from build123d import *

# Parameters (mm, degrees)
SKETCH1_R           = 10
BOSS_EXTRUDE1_DEPTH = 20
BOSS_EXTRUDE2_DEPTH = 20
CUT_EXTRUDE1_DEPTH  = 15
SKETCH5_R           = 20
BOSS_EXTRUDE3_DEPTH = 5


with BuildPart() as part:
    # Sketch1 → Boss-Extrude1 (new body)
    with BuildSketch(Plane.XY):
        with BuildLine():
            Line((-71.370560529, 20), (276.629439471, 20))
            ThreePointArc((276.629439471, 20), (296.629439471, 0), (276.629439471, -20))
            Line((276.629439471, -20), (-71.370560529, -20))
            ThreePointArc((-71.370560529, -20), (-91.370560529, 0), (-71.370560529, 20))
        make_face()
        with Locations((-71.370560529, 0)):
            Circle(SKETCH1_R, mode=Mode.SUBTRACT)
        with Locations((276.629439471, 0)):
            Circle(SKETCH1_R, mode=Mode.SUBTRACT)
    extrude(amount=BOSS_EXTRUDE1_DEPTH)

    # Sketch2 → Boss-Extrude2 (add)
    with BuildSketch(Plane(origin=(0, 0, 0), x_dir=(-1, 0, 0), z_dir=(0, 0, -1))):
        with BuildLine():
            Line((71.370560529, -20), (71.370560529, -25))
            ThreePointArc((71.370560529, -25), (64.900084402, -24.148145657), (58.870560529, -21.650635095))
            Line((58.870560529, -21.650635095), (62.564306071, -17.956889553))
            ThreePointArc((62.564306071, -17.956889553), (66.850482602, -19.482527955), (71.370560529, -20))
        make_face()
    extrude(amount=BOSS_EXTRUDE2_DEPTH)

    # Sketch6 → Cut-Extrude1 (cut)
    with BuildSketch(Plane.XY.offset(20)):
        with BuildLine():
            ThreePointArc((-88.39401573, 13.427541495), (-86.445115044, 11.855559488), (-84.410885886, 10.395678313))
            ThreePointArc((-84.410885886, 10.395678313), (-82.694985814, 12.298884863), (-80.712431568, 13.922457124))
            ThreePointArc((-80.712431568, 13.922457124), (-81.560998495, 16.374699705), (-82.281198511, 18.867664093))
            ThreePointArc((-82.281198511, 18.867664093), (-79.798448631, 20.149575363), (-77.17323964, 21.106456352))
            ThreePointArc((-77.17323964, 21.106456352), (-76.520533705, 18.689161112), (-75.73290437, 16.312402533))
            ThreePointArc((-75.73290437, 16.312402533), (-73.22603531, 16.843548219), (-70.667803401, 16.991729622))
            ThreePointArc((-70.667803401, 16.991729622), (-69.912916442, 19.47441067), (-69.030242792, 21.914584175))
            ThreePointArc((-69.030242792, 21.914584175), (-66.268167407, 21.492348412), (-63.581888186, 20.723422265))
            ThreePointArc((-63.581888186, 20.723422265), (-64.474688485, 18.384138413), (-65.234506609, 15.998343424))
            ThreePointArc((-65.234506609, 15.998343424), (-62.894207335, 14.954548647), (-60.737455402, 13.570738932))
            ThreePointArc((-60.737455402, 13.570738932), (-58.667455717, 15.135558669), (-56.519059735, 16.59087795))
            ThreePointArc((-56.519059735, 16.59087795), (-54.532677763, 14.625774866), (-52.811395672, 12.424745236))
            ThreePointArc((-52.811395672, 12.424745236), (-54.908682835, 11.056999694), (-56.925723719, 9.57346089))
            ThreePointArc((-56.925723719, 9.57346089), (-55.645909011, 7.353419778), (-54.714442987, 4.966187222))
            ThreePointArc((-54.714442987, 4.966187222), (-52.120000099, 5.015437696), (-49.526496029, 4.930020252))
            ThreePointArc((-49.526496029, 4.930020252), (-49.074537869, 2.172652432), (-48.97572416, -0.619762172))
            ThreePointArc((-48.97572416, -0.619762172), (-51.476405776, -0.493537095), (-53.98022836, -0.508158314))
            ThreePointArc((-53.98022836, -0.508158314), (-54.249743937, -3.056465513), (-54.899352183, -5.535279212))
            ThreePointArc((-54.899352183, -5.535279212), (-52.771455094, -7.020410009), (-50.72347334, -8.613937617))
            ThreePointArc((-50.72347334, -8.613937617), (-51.978571647, -11.110349384), (-53.539969801, -13.427541495))
            ThreePointArc((-53.539969801, -13.427541495), (-55.488870486, -11.855559488), (-57.523099645, -10.395678313))
            ThreePointArc((-57.523099645, -10.395678313), (-59.238999716, -12.298884863), (-61.221553963, -13.922457124))
            ThreePointArc((-61.221553963, -13.922457124), (-60.372987036, -16.374699705), (-59.65278702, -18.867664093))
            ThreePointArc((-59.65278702, -18.867664093), (-62.1355369, -20.149575363), (-64.760745891, -21.106456352))
            ThreePointArc((-64.760745891, -21.106456352), (-65.413451825, -18.689161112), (-66.20108116, -16.312402533))
            ThreePointArc((-66.20108116, -16.312402533), (-68.707950221, -16.843548219), (-71.26618213, -16.991729622))
            ThreePointArc((-71.26618213, -16.991729622), (-72.021069089, -19.47441067), (-72.903742738, -21.914584175))
            ThreePointArc((-72.903742738, -21.914584175), (-75.665818123, -21.492348412), (-78.352097344, -20.723422265))
            ThreePointArc((-78.352097344, -20.723422265), (-77.459297045, -18.384138413), (-76.699478922, -15.998343424))
            ThreePointArc((-76.699478922, -15.998343424), (-79.039778195, -14.954548647), (-81.196530129, -13.570738932))
            ThreePointArc((-81.196530129, -13.570738932), (-83.266529813, -15.135558669), (-85.414925795, -16.59087795))
            ThreePointArc((-85.414925795, -16.59087795), (-87.401307767, -14.625774866), (-89.122589859, -12.424745236))
            ThreePointArc((-89.122589859, -12.424745236), (-87.025302696, -11.056999694), (-85.008261811, -9.57346089))
            ThreePointArc((-85.008261811, -9.57346089), (-86.28807652, -7.353419778), (-87.219542544, -4.966187222))
            ThreePointArc((-87.219542544, -4.966187222), (-89.813985431, -5.015437696), (-92.407489502, -4.930020252))
            ThreePointArc((-92.407489502, -4.930020252), (-92.859447662, -2.172652432), (-92.95826137, 0.619762172))
            ThreePointArc((-92.95826137, 0.619762172), (-90.457579755, 0.493537095), (-87.953757171, 0.508158314))
            ThreePointArc((-87.953757171, 0.508158314), (-87.684241594, 3.056465513), (-87.034633347, 5.535279212))
            ThreePointArc((-87.034633347, 5.535279212), (-89.162530436, 7.020410009), (-91.210512191, 8.613937617))
            ThreePointArc((-91.210512191, 8.613937617), (-89.955413884, 11.110349384), (-88.39401573, 13.427541495))
        make_face()
    extrude(amount=-CUT_EXTRUDE1_DEPTH, mode=Mode.SUBTRACT)

    # Sketch5 → Boss-Extrude3 (add)
    with BuildSketch(Plane.XY.offset(15)):
        with Locations((-72.002203934, 0)):
            Circle(SKETCH5_R)
    extrude(amount=BOSS_EXTRUDE3_DEPTH)


solid = part.part
Input: part model. Units: mm. Frame: model coordinates. A direction names the side the tool comes from. Round coordinates to 2 decimals unless told otherwise and drop trailing zeros. Loops run counter-clockwise (first coordinate to the right, second up) from the corner with the lowest first, then second, coordinate; pieces in that order, holes last. Notation, with made-up numbers: (46, -14.75) -> (88, -14.75) arc R14 ccw to (88, 8.25) -> close; hole circle Ø9 at (58, 8.5). An arc over 180 degrees is marked (long way). Answer as a JSON object with one key per item and string values. Group by question number.
1) Section query A-A on z = 10.5. State how many separate pieces and enclosed holes the cut face has, plus the area to 3 significant figures.
2) Section query B-B on z = -16. Output: boundary loops of the cut face in (x, y), plus the area to 3 significant figures.
3) Draft query along Y for faces 1 (the flat face through (-65, -21, -20)), 2 (the flat face through (105, -20, 10)), 3 (the flat face through (-72, 0, 15)). Return one class per face: +Y half, -Y half, draft (parallel to the pull), parting line (faces both ways), or undercut.
4) Pin query (flat end, axial travel): pin 1 (6 mm diameter, centred on x = 101.5, z = 12.5, fed in from -Y); pin 2 (18 mm diameter, centred on x = 276.63, y = 0, fed in from +Z); pin 3 (3 mm diameter, centred on y = 10, z = 11, fed in from -X); pin 4 (2.5 mm diameter, centred on y = -21.5, z = -6.5, fed in from -X). Return the tip coordinate at first contact, or that it passes through.
5) Ray query, L1, parallel to X at y = 6, z = 14.5; L2, parallel to Y at x = 93, z = 18.5; L3, parallel to X at y = 11.5, z = 10.5. Return the intervals inside material, ascending.
6) Section query C-C on x = -24. Output: boundary loops of the cut face in (y, z), plus the area to 3 significant figures.
7) Reachability of faces 4 (the flat face through (-60, 0, 5)), 5 (the cylindrical face through (-66.79, -19.47, -9.86)), 6 (the flat face through (100, 20, 10)), 7 (the cylindrical face through (-61.83, 3, 2.46)), 8 (the cylindrical face through (-90.31, 6.43, 7.64)) from +Z, -Z, +X, -X, +Y, -Y: full face, straight path, thin tool, end or side. Return the list, or none.
Reply:
{
 "1": {"separate pieces": "7", "enclosed holes": "1", "area": "13,700 mm2"},
 "2": {"outline": "(-71.37, -25) arc R25 ccw to (-58.87, -21.65) -> (-62.56, -17.96) arc R20 cw to (-71.37, -20) -> close", "area": "55.5 mm2"},
 "3": {"face 1": "draft", "face 2": "-Y half", "face 3": "undercut"},
 "4": {"pin 1": "stops at y = -20", "pin 2": "passes through", "pin 3": "stops at x = -85.97", "pin 4": "stops at x = -71.37"},
 "5": {"L1": "x = -90.45 to -87.73, -55.07 to 268.63, 284.63 to 295.71", "L2": "y = -20 to 20", "L3": "x = -85.97 to -83.48, -54.26 to 292.99"},
 "6": {"outline": "(-20, 0) -> (20, 0) -> (20, 20) -> (-20, 20) -> close", "area": "800 mm2"},
 "7": {"face 4": "none", "face 5": "-Z, -X, +Y", "face 6": "+Z, -Z, +X, -X, +Y", "face 7": "-Z", "face 8": "-Z, -X"}
}
